from build123d import *

# Parameters (mm, degrees)
F1_W     = 460
F1_H     = 650
F2_DEPTH = 1500
F3_W     = 560
F3_H     = 750
F3_W_2   = 460
F3_H_2   = 650
F4_DEPTH = 100
F5_T     = -5
F6_R     = 100
F7_DEPTH = 50
F9_DEPTH = 50


with BuildPart() as f2:
    # F1 (on offset) → F2 (new body)
    with BuildSketch(Plane.XY.offset(50)):
        with Locations((280, 375)):
            Rectangle(F1_W, F1_H)
    extrude(amount=F2_DEPTH)

    # F3 (on face) → F4 (join)
    with BuildSketch(Plane.XY.offset(1550)):
        with Locations((280, 375)):
            Rectangle(F3_W, F3_H)
        with Locations((280, 375)):
            Rectangle(F3_W_2, F3_H_2, mode=Mode.SUBTRACT)
    extrude(amount=-F4_DEPTH)

    # F5
    f5_openings = [f2.faces().sort_by_distance(p)[0] for p in [
        (280, 375, 1550),
    ]]
    offset(amount=F5_T, openings=f5_openings, kind=Kind.INTERSECTION)

    # F6 (on Right) → F7 (join, through all)
    with BuildSketch(Plane.YZ):
        with Locations((650, 100)):
            Circle(F6_R)
    extrude(amount=F7_DEPTH)

    # F8 (on face) → F9 (join, through all)
    with BuildSketch(Plane.YZ.offset(510)):
        with BuildLine():
            ThreePointArc((563.3974596216, 50), (675.8819045103, 3.4074173711), (750, 100))
            ThreePointArc((750, 100), (736.6025403784, 150), (700, 186.6025403784))
            Line((700, 186.6025403784), (700, 50))
            Line((700, 50), (563.3974596216, 50))
        make_face()
        with BuildLine():
            Line((700, 50), (700, 186.6025403784))
            ThreePointArc((700, 186.6025403784), (579.2893218813, 170.7106781187), (563.3974596216, 50))
            Line((563.3974596216, 50), (700, 50))
        make_face()
    extrude(amount=F9_DEPTH)


solid = f2.part
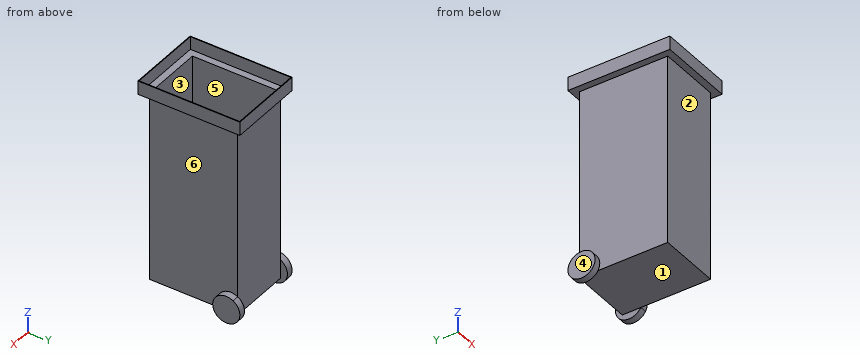
Geometry: final body of the model. Coordinates: model frame, mm. Face numbers are marked on the shaded views. A direction names the side the tool comes from. Give positions to 0.01 mm unless a question says otherwise; leave off trailing zeros. Order: outer loops, then holes, each group sorted by start corner. A loop starts at its lowest first (then second) coordinate and runs counter-clockwise, first axis right, second up. Notation, with made-up numbers: (-3, 75.5) -> (2, 75.5) arc R23 cw to (2, 114.5) -> close; hole circle Ø10 at (-18, 16.25). An arc over 180 degrees is marked (long way). Put each result on its own line as item: value.
Q1. Material intervals for L1, parallel to X at y = 154, z = 1108; L2, parallel to Y at x = 114.5, z = 1340.5; L3, parallel to Z at x = 277.5, y = 646, sorted ascending.
Here are the results:
L1: x = 50 to 55, 505 to 510
L2: y = 50 to 55, 695 to 700
L3: z = 50 to 55
Q2. Reachability of the marked faces 1, 2 and 3 from +Z, -Z, +X, -X, +Y, -Y: full face, straight path, thin tool, end or side. Return the list, or none.
Here are the results:
face 1: -Z, +Y, -Y
face 2: -Z, +X, -X, -Y
face 3: +Z
Q3. Section C-C, the plane x = 340.5. Return loops of the section in (y, z), then the cut area to 3 significant figures.
Here are the results:
outline: (0, 1450) -> (50, 1450) -> (50, 50) -> (700, 50) -> (700, 1450) -> (750, 1450) -> (750, 1550) -> (745, 1550) -> (745, 1455) -> (695, 1455) -> (695, 55) -> (55, 55) -> (55, 1455) -> (5, 1455) -> (5, 1550) -> (0, 1550) -> close
area: 18,700 mm^2
Q4. Section D-D, the plane z = 100. Return loops of the section in (x, y).
Here are the results:
outline: (0, 550) -> (50, 550) -> (50, 50) -> (510, 50) -> (510, 550) -> (560, 550) -> (560, 750) -> (510, 750) -> (510, 700) -> (50, 700) -> (50, 750) -> (0, 750) -> close; hole (55, 55) -> (505, 55) -> (505, 695) -> (55, 695) -> close
Q5. Pin query (flat end, axial travel): pin 1 (10 mm diameter, centred on y = 344, z = 186, fed in from -X); pin 2 (8 mm diameter, centred on y = 217, z = 1187, fed in from +X); pin 3 (8 mm diameter, centred on x = 152, z = 569, fed in from +Y). Return the tip coordinate at first contact, or that it passes through.
Here are the results:
pin 1: stops at x = 50
pin 2: stops at x = 510
pin 3: stops at y = 700
Q6. Draft query along X for the marked faces 4, 5 and 6. Return one class per face: released by +X, released by -X, zero draft, split by the parting line, or undercut.
Here are the results:
face 4: released by -X
face 5: undercut
face 6: released by +X
Q7. Section B-B, the plane y = 650. Return loops of the section in (x, z), then the cut area to 4 significant figures.
Here are the results:
outline: (0, 0) -> (50, 0) -> (50, 50) -> (510, 50) -> (510, 0) -> (560, 0) -> (560, 200) -> (510, 200) -> (510, 1450) -> (560, 1450) -> (560, 1550) -> (555, 1550) -> (555, 1455) -> (505, 1455) -> (505, 55) -> (55, 55) -> (55, 1455) -> (5, 1455) -> (5, 1550) -> (0, 1550) -> (0, 1450) -> (50, 1450) -> (50, 200) -> (0, 200) -> close
area: 37,750 mm^2
Q8. Section A-A, the plane z = 597. Return loops of the section in (x, y), then the cut area to 3 significant figures.
Here are the results:
outline: (50, 50) -> (510, 50) -> (510, 700) -> (50, 700) -> close; hole (55, 55) -> (505, 55) -> (505, 695) -> (55, 695) -> close
area: 11,000 mm^2
